```python
from build123d import *

# Parameters (mm, degrees)
SKETCH1_R           = 5
BOSS_EXTRUDE1_DEPTH = 2.5
SKETCH2_R           = 6.25
BOSS_EXTRUDE2_DEPTH = 3.5
SKETCH3_R           = 4
CUT_EXTRUDE1_DEPTH  = 7.5
SKETCH4_R           = 5
CUT_EXTRUDE2_DEPTH  = 2.5


with BuildPart() as part:
    # Sketch1 → Boss-Extrude1 (new body)
    with BuildSketch(Plane(origin=(0, 0, 0), x_dir=(1, 0, 0), z_dir=(0, 1, 0))):
        Circle(SKETCH1_R)
    extrude(amount=BOSS_EXTRUDE1_DEPTH)

    # Sketch2 → Boss-Extrude2 (add)
    with BuildSketch(Plane.XZ):
        Circle(SKETCH2_R)
    extrude(amount=BOSS_EXTRUDE2_DEPTH)

    # Sketch3 → Cut-Extrude1 (cut)
    with BuildSketch(Plane(origin=(0, 2.5, 0), x_dir=(1, 0, 0), z_dir=(0, 1, 0))):
        Circle(SKETCH3_R)
    extrude(amount=-CUT_EXTRUDE1_DEPTH, mode=Mode.SUBTRACT)

    # Sketch4 → Cut-Extrude2 (cut)
    with BuildSketch(Plane.XZ.offset(3.5)):
        Circle(SKETCH4_R)
    extrude(amount=-CUT_EXTRUDE2_DEPTH, mode=Mode.SUBTRACT)


solid = part.part
```
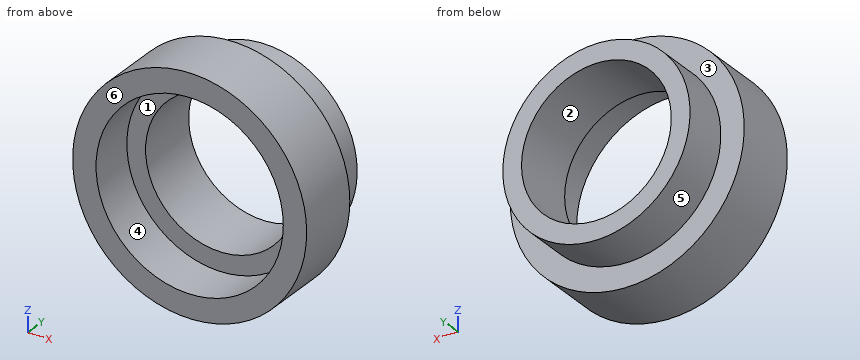
For this review, take the finished solid that the model builds, in its own axes (mm). Face numbers are marked on the shaded views. A direction names the side the tool comes from. Give positions to 0.01 mm unless a question says otherwise; leave off trailing zeros. Write each loop counter-clockwise with the first axis right and the second up, starting at its lowest first coordinate (ties: lowest second). Pieces come first, ordered by that corner, then holes. Notation, with made-up numbers: M -7.5,-17 L 39.5,-17 A28 ccw 39.5,4 Z; hole C 37,39 d9. An arc over 180 degrees is marked long. Answer as a JSON object with one key per item and string values. Group by question number.
Item 1: Draft analysis for pull direction X (two halves, no side actions). For the marked faces 4, 5 and 6, state which applies: +X half, -X half, draft (parallel to the pull), parting line (faces both ways), or undercut.
Item 2: Consider section B-B on z = 0. Write out the cut boundary in (x, y).
Item 3: Consider section C-C on y = -1.65. Write out the cut boundary in (x, z).
Item 4: Consider section D-D on x = -4.75. Write out the cut boundary in (y, z), plus the area to 3 significant figures.
Item 5: For pin 1 Ø1 at (y, z) = (1, 2.5) entering from -X; pin 2 Ø1 at (x, y) = (-4, -1) entering from +Z; pin 3 Ø6.5 at (x, z) = (0, 0) entering from -Y, all flat-tipped, find the tip position at first contact; note any pin that passes through.
Item 6: Consider section A-A on x = 0. Write out the cut boundary in (y, z), plus the area to 4 significant figures.
Item 7: For probe 1 along Z at (x, y) = (0, 0.8); probe 2 along Z at (x, y) = (0, -2.4); probe 3 along X at (y, z) = (1.7, 3), list the stretches that pass through material, from the lowest coordinate up. Write a range as [from, to].
Item 8: Tool access review of the marked faces 1, 2 and 3: name each direction out of +Z, -Z, +X, -X, +Y, -Y from which nothing blocks a thin tool from reaching the whole face with its end or side.
Check result:
{
 "1": {"face 4": "undercut", "face 5": "parting line", "face 6": "draft"},
 "2": {"outline": "M -6.25,-3.5 L -5,-3.5 L -5,-1 L -4,-1 L -4,2.5 L -5,2.5 L -5,0 L -6.25,0 Z; M 4,-1 L 5,-1 L 5,-3.5 L 6.25,-3.5 L 6.25,0 L 5,0 L 5,2.5 L 4,2.5 Z"},
 "3": {"outline": "C 0,0 d12.5; hole C 0,0 d10"},
 "4": {"outline": "M -3.5,-4.06 L 0,-4.06 L 0,-1.56 L 2.5,-1.56 L 2.5,1.56 L 0,1.56 L 0,4.06 L -3.5,4.06 L -3.5,1.56 L -1,1.56 L -1,-1.56 L -3.5,-1.56 Z", "area": "28.4 mm^2"},
 "5": {"pin 1": "stops at x = -4.58", "pin 2": "stops at z = 5.18", "pin 3": "passes through"},
 "6": {"outline": "M -3.5,-6.25 L 0,-6.25 L 0,-5 L 2.5,-5 L 2.5,-4 L -1,-4 L -1,-5 L -3.5,-5 Z; M -3.5,5 L -1,5 L -1,4 L 2.5,4 L 2.5,5 L 0,5 L 0,6.25 L -3.5,6.25 Z", "area": "15.75 mm^2"},
 "7": {"probe 1": "z = [-5, -4], [4, 5]", "probe 2": "z = [-6.25, -5], [5, 6.25]", "probe 3": "x = [-4, -2.65], [2.65, 4]"},
 "8": {"face 1": "-Y", "face 2": "+Y, -Y", "face 3": "+Y"}
}
